```python
from build123d import *

# Parameters (mm, degrees)
SKETCH_1_W      = 45
SKETCH_1_H      = 45
SKETCH_1_R      = 1.5
SKETCH_1_R_2    = 20
EXTRUDE_1_DEPTH = 10
SKETCH_2_R      = 20
EXTRUDE_2_DEPTH = 1


with BuildPart() as part:
    # 草圖1 → 填料-伸長1 (new body)
    with BuildSketch(Plane.XY):
        Rectangle(SKETCH_1_W, SKETCH_1_H)
        with Locations((19, 19)):
            Circle(SKETCH_1_R, mode=Mode.SUBTRACT)
        with Locations((19, -19)):
            Circle(SKETCH_1_R, mode=Mode.SUBTRACT)
        with Locations((-19, -19)):
            Circle(SKETCH_1_R, mode=Mode.SUBTRACT)
        Circle(SKETCH_1_R_2, mode=Mode.SUBTRACT)
    extrude(amount=EXTRUDE_1_DEPTH)

    # 草圖2 → 填料-伸長2 (add)
    with BuildSketch(Plane(origin=(0, 0, 0), x_dir=(-1, 0, 0), z_dir=(0, 0, -1))):
        Circle(SKETCH_2_R)
    extrude(amount=-EXTRUDE_2_DEPTH)


solid = part.part
```
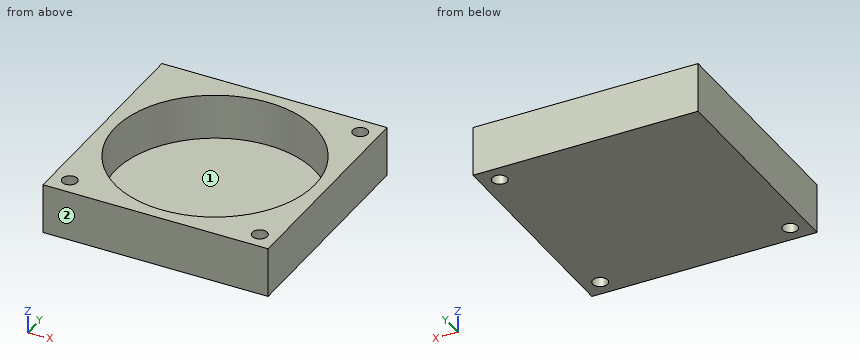
Verification items for the finished model (mm, model axes). Face numbers are marked on the shaded views. A direction names the side the tool comes from. Round coordinates to 2 decimals unless told otherwise and drop trailing zeros. Write each loop counter-clockwise with the first axis right and the second up, starting at its lowest first coordinate (ties: lowest second). Pieces come first, ordered by that corner, then holes.
1. Section check A-A on y = 0. Enter the section's corners in (x, z), plus the area to 3 significant figures.
2. Section check C-C on x = 19. Enter the section's corners in (y, z) (3 decimals), plus the area to 3 significant figures.
3. Access from +Z, -Z, +X, -X, +Y, -Y to the whole of each face (thin tool, end or side, straight path). Record for the marked faces 1 and 2.
4. Section check B-B on z = 2.75. Enter the section's corners in (x, y), plus the area to 3 significant figures.
5. Gauge pin test, flat ends, axial feed: P1, Ø10, axis at x = -5.5, y = 13.5, coming from the +Z side; P2, Ø2.5, axis at x = 19, y = 19, coming from the +Z side. Record the tip position at first contact, or that the pin passes through.
6. Scan lines: L1, parallel to Y at x = 0, z = 3.25; L2, parallel to Y at x = 4.5, z = 6.75. Record each from-to range of solid material in increasing order.
Answer:
1. outline: (-22.5, 0) - (22.5, 0) - (22.5, 10) - (20, 10) - (20, 1) - (-20, 1) - (-20, 10) - (-22.5, 10) - close
1. area: 90.0 mm2
2. outline: (-22.5, 0) - (-20.5, 0) - (-20.5, 10) - (-22.5, 10) - close; (-17.5, 0) - (17.5, 0) - (17.5, 10) - (6.245, 10) - (6.245, 1) - (-6.245, 1) - (-6.245, 10) - (-17.5, 10) - close; (20.5, 0) - (22.5, 0) - (22.5, 10) - (20.5, 10) - close
2. area: 278 mm2
3. face 1: +Z
3. face 2: +Z, -Z, +X, -X, -Y
4. outline: (-22.5, -22.5) - (22.5, -22.5) - (22.5, 22.5) - (-22.5, 22.5) - close; hole circle Ø3 at (-19, -19); hole circle Ø40 at (0, 0); hole circle Ø3 at (19, -19); hole circle Ø3 at (19, 19)
4. area: 747 mm2
5. P1: stops at z = 1
5. P2: passes through
6. L1: y = -22.5 to -20, 20 to 22.5
6. L2: y = -22.5 to -19.49, 19.49 to 22.5
